Geometry: final body of the model. Coordinates: model frame, mm. A direction names the side the tool comes from. Give positions to 0.01 mm unless a question says otherwise; leave off trailing zeros. Write each loop counter-clockwise with the first axis right and the second up, starting at its lowest first coordinate (ties: lowest second). Pieces come first, ordered by that corner, then holes. Notation, with made-up numbers: (53.25, 52) -> (108.25, 52) arc R8 cw to (108.25, 63) -> close; hole circle Ø4 at (82, 34.5). An arc over 180 degrees is marked (long way). Answer as a JSON object with one key per item and string values.
from build123d import *

# Parameters (mm, degrees)
SKETCH_W          = 220
SKETCH_H          = 220
PAD_DEPTH         = 10
BOX_W             = 188
BOX_H             = 95
BOX_DEPTH         = 25
BOX001_W          = 186
BOX001_H          = 93
BOX001_DEPTH      = 20
BOX002_W          = 150
BOX002_H          = 95
BOX002_DEPTH      = 20
CYLINDER_R        = 18
CYLINDER_DEPTH    = 60
CYLINDER001_R     = 17
CYLINDER001_DEPTH = 60
CYLINDER002_R     = 16
CYLINDER002_DEPTH = 60
CYLINDER003_R     = 17
CYLINDER003_DEPTH = 60
CYLINDER004_R     = 16
CYLINDER004_DEPTH = 60
CYLINDER005_R     = 17
CYLINDER005_DEPTH = 60
CYLINDER006_R     = 16
CYLINDER006_DEPTH = 60
CYLINDER007_R     = 17
CYLINDER007_DEPTH = 60
CYLINDER008_R     = 16
CYLINDER008_DEPTH = 60
CYLINDER009_R     = 16
CYLINDER009_DEPTH = 60
CYLINDER010_R     = 17
CYLINDER010_DEPTH = 60
CYLINDER011_R     = 16
CYLINDER011_DEPTH = 60
CYLINDER012_R     = 17
CYLINDER012_DEPTH = 60
CYLINDER013_R     = 16
CYLINDER013_DEPTH = 60
CYLINDER014_R     = 26
CYLINDER014_DEPTH = 60
CYLINDER015_R     = 25
CYLINDER015_DEPTH = 60
CYLINDER016_R     = 26
CYLINDER016_DEPTH = 60
CYLINDER017_R     = 25
CYLINDER017_DEPTH = 60


with BuildPart() as part:
    # Sketch → Pad (new body)
    with BuildSketch(Plane.XY):
        Rectangle(SKETCH_W, SKETCH_H)
    extrude(amount=PAD_DEPTH)

    # Box → Box (join)
    with BuildSketch(Plane(origin=(-92, 4, 10), x_dir=(1, 0, 0), z_dir=(0, 0, 1))):
        with Locations((94, 47.5)):
            Rectangle(BOX_W, BOX_H)
    extrude(amount=BOX_DEPTH)

    # Box001 → Box001 (cut)
    with BuildSketch(Plane(origin=(-91, 5, 20), x_dir=(1, 0, 0), z_dir=(0, 0, 1))):
        with Locations((93, 46.5)):
            Rectangle(BOX001_W, BOX001_H)
    extrude(amount=BOX001_DEPTH, mode=Mode.SUBTRACT)

    # Box002 → Box002 (cut)
    with BuildSketch(Plane(origin=(-75, 4, 20), x_dir=(1, 0, 0), z_dir=(0, 0, 1))):
        with Locations((75, 47.5)):
            Rectangle(BOX002_W, BOX002_H)
    extrude(amount=BOX002_DEPTH, mode=Mode.SUBTRACT)

    # Cylinder → Cylinder (join)
    with BuildSketch(Plane(origin=(0, -20, 10), x_dir=(1, 0, 0), z_dir=(0, 0, 1))):
        Circle(CYLINDER_R)
    extrude(amount=CYLINDER_DEPTH)

    # Cylinder001 → Cylinder001 (join)
    with BuildSketch(Plane(origin=(40, -20, 10), x_dir=(1, 0, 0), z_dir=(0, 0, 1))):
        Circle(CYLINDER001_R)
    extrude(amount=CYLINDER001_DEPTH)

    # Cylinder002 → Cylinder002 (cut)
    with BuildSketch(Plane(origin=(40, -20, 10), x_dir=(1, 0, 0), z_dir=(0, 0, 1))):
        Circle(CYLINDER002_R)
    extrude(amount=CYLINDER002_DEPTH, mode=Mode.SUBTRACT)

    # Cylinder003 → Cylinder003 (join)
    with BuildSketch(Plane(origin=(80, -20, 10), x_dir=(1, 0, 0), z_dir=(0, 0, 1))):
        Circle(CYLINDER003_R)
    extrude(amount=CYLINDER003_DEPTH)

    # Cylinder004 → Cylinder004 (cut)
    with BuildSketch(Plane(origin=(80, -20, 10), x_dir=(1, 0, 0), z_dir=(0, 0, 1))):
        Circle(CYLINDER004_R)
    extrude(amount=CYLINDER004_DEPTH, mode=Mode.SUBTRACT)

    # Cylinder005 → Cylinder005 (join)
    with BuildSketch(Plane(origin=(-40, -20, 10), x_dir=(1, 0, 0), z_dir=(0, 0, 1))):
        Circle(CYLINDER005_R)
    extrude(amount=CYLINDER005_DEPTH)

    # Cylinder006 → Cylinder006 (cut)
    with BuildSketch(Plane(origin=(-40, -20, 10), x_dir=(1, 0, 0), z_dir=(0, 0, 1))):
        Circle(CYLINDER006_R)
    extrude(amount=CYLINDER006_DEPTH, mode=Mode.SUBTRACT)

    # Cylinder007 → Cylinder007 (join)
    with BuildSketch(Plane(origin=(-80, -20, 10), x_dir=(1, 0, 0), z_dir=(0, 0, 1))):
        Circle(CYLINDER007_R)
    extrude(amount=CYLINDER007_DEPTH)

    # Cylinder008 → Cylinder008 (cut)
    with BuildSketch(Plane(origin=(-80, -20, 10), x_dir=(1, 0, 0), z_dir=(0, 0, 1))):
        Circle(CYLINDER008_R)
    extrude(amount=CYLINDER008_DEPTH, mode=Mode.SUBTRACT)

    # Cylinder009 → Cylinder009 (cut)
    with BuildSketch(Plane(origin=(0, -20, 10), x_dir=(1, 0, 0), z_dir=(0, 0, 1))):
        Circle(CYLINDER009_R)
    extrude(amount=CYLINDER009_DEPTH, mode=Mode.SUBTRACT)

    # Cylinder010 → Cylinder010 (join)
    with BuildSketch(Plane(origin=(-79, -65, 10), x_dir=(1, 0, 0), z_dir=(0, 0, 1))):
        Circle(CYLINDER010_R)
    extrude(amount=CYLINDER010_DEPTH)

    # Cylinder011 → Cylinder011 (cut)
    with BuildSketch(Plane(origin=(-79, -65, 10), x_dir=(1, 0, 0), z_dir=(0, 0, 1))):
        Circle(CYLINDER011_R)
    extrude(amount=CYLINDER011_DEPTH, mode=Mode.SUBTRACT)

    # Cylinder012 → Cylinder012 (join)
    with BuildSketch(Plane(origin=(-39, -65, 10), x_dir=(1, 0, 0), z_dir=(0, 0, 1))):
        Circle(CYLINDER012_R)
    extrude(amount=CYLINDER012_DEPTH)

    # Cylinder013 → Cylinder013 (cut)
    with BuildSketch(Plane(origin=(-39, -65, 10), x_dir=(1, 0, 0), z_dir=(0, 0, 1))):
        Circle(CYLINDER013_R)
    extrude(amount=CYLINDER013_DEPTH, mode=Mode.SUBTRACT)

    # Cylinder014 → Cylinder014 (join)
    with BuildSketch(Plane(origin=(11, -70, 10), x_dir=(1, 0, 0), z_dir=(0, 0, 1))):
        Circle(CYLINDER014_R)
    extrude(amount=CYLINDER014_DEPTH)

    # Cylinder015 → Cylinder015 (cut)
    with BuildSketch(Plane(origin=(11, -70, 10), x_dir=(1, 0, 0), z_dir=(0, 0, 1))):
        Circle(CYLINDER015_R)
    extrude(amount=CYLINDER015_DEPTH, mode=Mode.SUBTRACT)

    # Cylinder016 → Cylinder016 (join)
    with BuildSketch(Plane(origin=(71, -70, 10), x_dir=(1, 0, 0), z_dir=(0, 0, 1))):
        Circle(CYLINDER016_R)
    extrude(amount=CYLINDER016_DEPTH)

    # Cylinder017 → Cylinder017 (cut)
    with BuildSketch(Plane(origin=(71, -70, 10), x_dir=(1, 0, 0), z_dir=(0, 0, 1))):
        Circle(CYLINDER017_R)
    extrude(amount=CYLINDER017_DEPTH, mode=Mode.SUBTRACT)


solid = part.part
Q1. Cut plane D-D (x = 40). Return the cut outline in (y, z).
Values:
{"outline": "(-110, 0) -> (110, 0) -> (110, 10) -> (99, 10) -> (99, 20) -> (4, 20) -> (4, 10) -> (-3, 10) -> (-3, 70) -> (-4, 70) -> (-4, 10) -> (-36, 10) -> (-36, 70) -> (-37, 70) -> (-37, 10) -> (-110, 10) -> close"}
Q2. Mould query, pull axis Y, two halves, no side actions, for faces 6 (the flat face through (-2, -110, 5)), 7 (the cylindrical face through (-42.213, -3.145, 39.58)), 8 (the flat face through (-39, -65, 10)), 9 (the flat face through (-66, -75, 70)). Classes: pulls with the +Y half, pulls with the -Y half, needs draft (parallel to the pull), parting line crosses it, or undercut.
Values:
{"face 6": "pulls with the -Y half", "face 7": "undercut", "face 8": "undercut", "face 9": "needs draft"}
Q3. Cut plane A-A (z = 53.5). State how many separate pieces and enclosed holes the cut face has, and give its area (3 significant figures).
Values:
{"separate pieces": "9", "enclosed holes": "9", "area": "1,160 mm²"}
Q4. Material intervals for L1, parallel to X at y = -92, z = 66; L2, parallel to Y at x = 71, z = 37.5; L3, parallel to Y at x = 54, z = 38, sorted ascending. Write a range as from..to.
Values:
{"L1": "-2.86..-0.87, 22.87..24.86, 57.14..59.13, 82.87..84.86", "L2": "-96..-95, -45..-44, -34.42..-33.23, -6.77..-5.58", "L3": "-89.67..-88.33, -51.67..-50.33, -29.64..-27.75, -12.25..-10.36"}
Q5. Cut plane C-C (y = 79.5). Return the cut outline in (x, z), and give its area (3 significant figures).
Values:
{"outline": "(-110, 0) -> (110, 0) -> (110, 10) -> (96, 10) -> (96, 35) -> (95, 35) -> (95, 20) -> (-91, 20) -> (-91, 35) -> (-92, 35) -> (-92, 10) -> (-110, 10) -> close", "area": "4,110 mm²"}
Q6. Set-up query: faces 1 (the flat face through (-2, 2, 0)), 2 (the flat face through (-29, -78, 70)), 3 (the flat face through (1, 4, 17)), 4 (the flat face through (-92, 51, 22)), 5 (the cylindrical face through (46.024, -68.901, 39.58)). Return all of +Z, -Z, +X, -X, +Y, -Y with unobstructed straight access to the full face (end or side cutting, diameter ignored); none if empty.
Values:
{"face 1": "-Z, +X, -X, +Y, -Y", "face 2": "+Z, +X, -X, +Y, -Y", "face 3": "+Z, +X, -X", "face 4": "+Z, -X, +Y", "face 5": "+Z"}
Q7. First-contact query: P1, Ø1.5, axis at y = -60, z = 57, coming from the +X side; P2, Ø4.5, axis at y = 54.5, z = 24, coming from the +X side; P3, Ø5, axis at y = 13, z = 23.5, coming from the -X side; P4, Ø8, axis at x = -24, z = 11, coming from the -Y side. Flat tips, straight axial feed; report the tip coordinate or a pass-through.
Values:
{"P1": "x = 95.3", "P2": "x = 96", "P3": "x = -92", "P4": "y = -110"}
